The model under review builds one solid part; all positions refer to its coordinate system, in mm. A direction names the side the tool comes from. Give positions to 0.01 mm unless a question says otherwise; leave off trailing zeros. Write each loop counter-clockwise with the first axis right and the second up, starting at its lowest first coordinate (ties: lowest second). Pieces come first, ordered by that corner, then holes. Notation, with made-up numbers: (-35, -31) -> (-25, -31) arc R13 cw to (-25, -9) -> close; hole circle Ø4 at (63, -26). An arc over 180 degrees is marked (long way). Use CSV: the item, a comma, the result in double quotes.
```python
from build123d import *

# Parameters (mm, degrees)
F0_R     = 12.7
F0_W     = 0.6285263425
F0_H     = 3.81
F1_DEPTH = 12.7
F2_DEPTH = 2.54
F0_R_2   = 6.477
F3_DEPTH = 27.94


# Not quite as in the source:
# - a feature names something its author has since deleted; it is built from what else it names


with BuildPart() as f1:
    # F0 (on Front) → F1 (new body)
    with BuildSketch(Plane.XZ):
        Circle(F0_R)
        Polygon((9.8425, 5.6825700245), (9.8425, 1.905), (10.4710263425, 1.905), (10.4710263425, -1.905), (9.8425, -1.905), (9.8425, -5.6825700245), (0, -11.365140049), (-9.8425, -5.6825700245), (-9.8425, -1.905), (-10.4710263425, -1.905), (-10.4710263425, 1.905), (-9.8425, 1.905), (-9.8425, 5.6825700245), (0, 11.365140049), align=None, mode=Mode.SUBTRACT)
        with Locations((10.1567631713, 0)):
            Rectangle(F0_W, F0_H)
        with Locations((-10.1567631713, 0)):
            Rectangle(F0_W, F0_H)
    extrude(amount=F1_DEPTH)

    # F0 (on Front) → F2 (join)
    with BuildSketch(Plane.XZ):
        Circle(F0_R)
        Polygon((9.8425, 5.6825700245), (9.8425, 1.905), (10.4710263425, 1.905), (10.4710263425, -1.905), (9.8425, -1.905), (9.8425, -5.6825700245), (0, -11.365140049), (-9.8425, -5.6825700245), (-9.8425, -1.905), (-10.4710263425, -1.905), (-10.4710263425, 1.905), (-9.8425, 1.905), (-9.8425, 5.6825700245), (0, 11.365140049), align=None, mode=Mode.SUBTRACT)
        with BuildLine():
            ThreePointArc((-7.2960263425, 1.905), (0, 7.540625), (7.2960263425, 1.905))
            Line((7.2960263425, 1.905), (9.8425, 1.905))
            Line((9.8425, 1.905), (9.8425, 5.6825700245))
            Line((9.8425, 5.6825700245), (0, 11.365140049))
            Line((0, 11.365140049), (-9.8425, 5.6825700245))
            Line((-9.8425, 5.6825700245), (-9.8425, 1.905))
            Line((-9.8425, 1.905), (-7.2960263425, 1.905))
        make_face()
        with BuildLine():
            Line((9.8425, -1.905), (7.2960263425, -1.905))
            ThreePointArc((7.2960263425, -1.905), (0, -7.540625), (-7.2960263425, -1.905))
            Line((-7.2960263425, -1.905), (-9.8425, -1.905))
            Line((-9.8425, -1.905), (-9.8425, -5.6825700245))
            Line((-9.8425, -5.6825700245), (0, -11.365140049))
            Line((0, -11.365140049), (9.8425, -5.6825700245))
            Line((9.8425, -5.6825700245), (9.8425, -1.905))
        make_face()
    extrude(amount=-F2_DEPTH)

    # F0 (on Front) → F3 (join)
    with BuildSketch(Plane.XZ):
        with BuildLine():
            ThreePointArc((7.2960263425, 1.905), (7.4792253619, 0.9603194134), (7.540625, 0))
            ThreePointArc((7.540625, 0), (7.4792253619, -0.9603194134), (7.2960263425, -1.905))
            Line((7.2960263425, -1.905), (9.8425, -1.905))
            Line((9.8425, -1.905), (9.8425, 1.905))
            Line((9.8425, 1.905), (7.2960263425, 1.905))
        make_face()
        with BuildLine():
            ThreePointArc((7.2960263425, -1.905), (7.4792253619, -0.9603194134), (7.540625, 0))
            ThreePointArc((7.540625, 0), (7.4792253619, 0.9603194134), (7.2960263425, 1.905))
            Line((7.2960263425, 1.905), (7.2960263425, -1.905))
        make_face()
        with BuildLine():
            Line((7.2960263425, -1.905), (7.2960263425, 1.905))
            ThreePointArc((7.2960263425, 1.905), (0, 7.540625), (-7.2960263425, 1.905))
            Line((-7.2960263425, 1.905), (-7.2960263425, -1.905))
            ThreePointArc((-7.2960263425, -1.905), (0, -7.540625), (7.2960263425, -1.905))
        make_face()
        Circle(F0_R_2, mode=Mode.SUBTRACT)
        with BuildLine():
            Line((-7.2960263425, -1.905), (-7.2960263425, 1.905))
            ThreePointArc((-7.2960263425, 1.905), (-7.540625, 0), (-7.2960263425, -1.905))
        make_face()
        with BuildLine():
            ThreePointArc((-7.2960263425, -1.905), (-7.540625, 0), (-7.2960263425, 1.905))
            Line((-7.2960263425, 1.905), (-9.8425, 1.905))
            Line((-9.8425, 1.905), (-9.8425, -1.905))
            Line((-9.8425, -1.905), (-7.2960263425, -1.905))
        make_face()
        with Locations((10.1567631713, 0)):
            Rectangle(F0_W, F0_H)
        with Locations((-10.1567631713, 0)):
            Rectangle(F0_W, F0_H)
    extrude(amount=-F3_DEPTH)


solid = f1.part
```
Q1. Consider section D-D (x = 8.5). Write out the cut boundary in (y, z) (3 decimals), then the cut area to 3 significant figures.
Derived:
outline,"(-12.7, -9.436) -> (2.54, -9.436) -> (2.54, -1.905) -> (27.94, -1.905) -> (27.94, 1.905) -> (2.54, 1.905) -> (2.54, 9.436) -> (-12.7, 9.436) -> (-12.7, 6.458) -> (0, 6.458) -> (0, -6.458) -> (-12.7, -6.458) -> close"
area,"220 mm2"
Q2. Consider section A-A (z = 0). Write out the cut boundary in (x, y), then the cut area to 3 significant figures.
Derived:
outline,"(-12.7, -12.7) -> (-9.84, -12.7) -> (-9.84, 0) -> (-6.48, 0) -> (-6.48, 27.94) -> (-10.47, 27.94) -> (-10.47, 2.54) -> (-12.7, 2.54) -> close; (6.48, 0) -> (9.84, 0) -> (9.84, -12.7) -> (12.7, -12.7) -> (12.7, 2.54) -> (10.47, 2.54) -> (10.47, 27.94) -> (6.48, 27.94) -> close"
area,"307 mm2"
Q3. To check wall thickness, follow probe 1 along Z at (x, y) = (0, 15.5); probe 2 along Z at (x, y) = (2.5, 15.5); probe 3 along Y at (x, z) = (-0.75, 8). State the ranges of each line that lie inside material, in increasing order.
Derived:
probe 1,"z = -7.54 to -6.48, 6.48 to 7.54"
probe 2,"z = -7.11 to -5.98, 5.98 to 7.11"
probe 3,"y = 0 to 2.54"
Q4. Insertion check: pin 1 (3 mm diameter, centred on x = 0, z = 9.5, fed in from -Y); pin 2 (1.9 mm diameter, centred on y = 16.5, z = 0.5, fed in from -X); pin 3 (4 mm diameter, centred on y = -2, z = 8, fed in from -X); pin 4 (6 mm diameter, centred on x = -1.5, z = 1.5, fed in from -Y). Each pin has a flat end and moves straight along its axis. Give the tip position at first contact, or say it passes through.
Derived:
pin 1,"stops at y = 0"
pin 2,"stops at x = -10.47"
pin 3,"stops at x = -11.19"
pin 4,"passes through"
Q5. Machinability: for faces 1 (the flat face through (4.852, -6.261, 8.564)), 2 (the flat face through (9, 15, 1.905)), 3 (the flat face through (9, 15, -1.905)), which of the approach directions +Z, -Z, +X, -X, +Y, -Y give a long, thin tool a straight path to every point of the face, cutting with its end or side? Answer none if there is none.
Derived:
face 1,"-Y"
face 2,"+Z, +X, +Y"
face 3,"-Z, +X, +Y"
Q6. The part is to be moulded in two halves that separate along Z. For faces 4 (the flat face through (-10.471, 15, 0)), 5 (the flat face through (9.842, -6, 0)), 6 (the cylindrical face through (-0.14, 15.06, -7.54)), say which applies: pulls with the +Z half, pulls with the -Z half, needs draft (parallel to the pull), parting line crosses it, or undercut.
Derived:
face 4,"needs draft"
face 5,"undercut"
face 6,"pulls with the -Z half"
Q7. Consider section C-C (x = -2.5). Write out the cut boundary in (y, z), then the cut area to 3 significant figures.
Derived:
outline,"(-12.7, -12.45) -> (2.54, -12.45) -> (2.54, -7.11) -> (27.94, -7.11) -> (27.94, -5.98) -> (0, -5.98) -> (0, -9.92) -> (-12.7, -9.92) -> close; (-12.7, 9.92) -> (0, 9.92) -> (0, 5.98) -> (27.94, 5.98) -> (27.94, 7.11) -> (2.54, 7.11) -> (2.54, 12.45) -> (-12.7, 12.45) -> close"
area,"155 mm2"
Q8. Consider section B-B (y = 23). Write out the cut boundary in (x, z) (3 decimals).
Derived:
outline,"(-10.471, -1.905) -> (-7.296, -1.905) arc R7.541 ccw to (7.296, -1.905) -> (10.471, -1.905) -> (10.471, 1.905) -> (7.296, 1.905) arc R7.541 ccw to (-7.296, 1.905) -> (-10.471, 1.905) -> close; hole circle Ø12.954 at (0, 0)"
